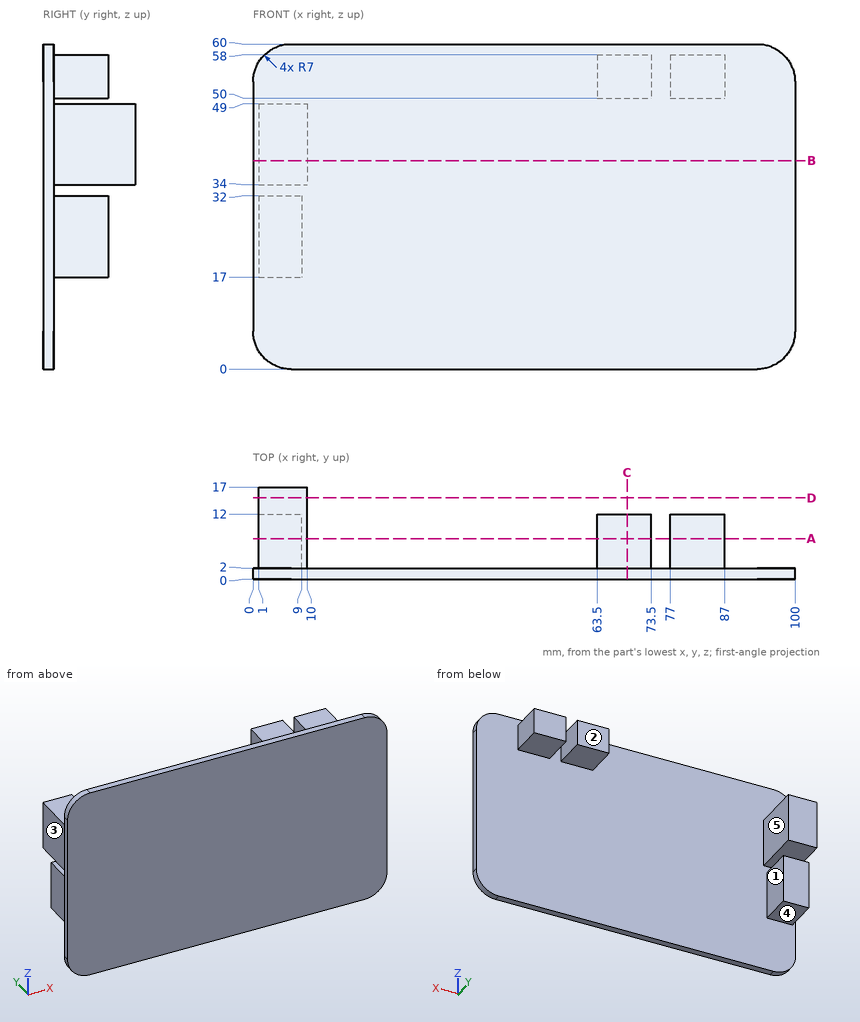
Geometry: see drawing. Coordinates: mm, zero at the bounding-box minimum. A direction names the side the tool comes from. Give positions to 0.01 mm unless a question says otherwise; leave off trailing zeros. Loops run counter-clockwise (first coordinate to the right, second up) from the corner with the lowest first, then second, coordinate; pieces in that order, holes last. Notation, with made-up numbers: (33, 55) -> (68, 55) arc R30 cw to (68, 83) -> close; hole circle Ø9 at (77, 0.25). An arc over 180 degrees is marked (long way). Put each result on its own line as item: value.
1. Set-up query: the marked faces 1, 2, 3, 4 and 5. Return all of +Z, -Z, +X, -X, +Y, -Y with unobstructed straight access to the full face (end or side cutting, diameter ignored); none if empty.
Taken from the geometry:
face 1: -Z, +X, +Y
face 2: +Z, -Z, +X, -X, +Y
face 3: +Z, -Z, -X, +Y
face 4: -Z, +X, -X, +Y
face 5: +Z, -Z, +X, +Y
2. Ray query, line 1 along Y through (x, z) = (17, 53.5); line 2 along X through (y, z) = (14.5, 44); line 3 along X through (y, z) = (11.5, 21). Return the intervals inside material, ascending. Write a range as [from, to].
Taken from the geometry:
line 1: y = [0, 2]
line 2: x = [1, 10]
line 3: x = [1, 9]
3. Cut plane C-C (x = 69). Return the cut outline in (y, z), plus the area to 3 significant figures.
Taken from the geometry:
outline: (0, 0) -> (2, 0) -> (2, 50) -> (12, 50) -> (12, 58) -> (2, 58) -> (2, 60) -> (0, 60) -> close
area: 200 mm2
4. Pin query (flat end, axial travel): P1, Ø7.5, axis at y = 7.5, z = 43.5, coming from the -X side; P2, Ø4, axis at x = 4.5, z = 21, coming from the +Y side; P3, Ø9, axis at x = 5, y = 9, coming from the +Z side; P4, Ø8, axis at x = 49.5, y = 9, coming from the -Z side. Return the tip coordinate at first contact, or that it passes through.
Taken from the geometry:
P1: stops at x = 1
P2: stops at y = 12
P3: stops at z = 49
P4: passes through
5. Cut plane B-B (z = 38.5). Return the cut outline in (x, y).
Taken from the geometry:
outline: (0, 0) -> (100, 0) -> (100, 2) -> (10, 2) -> (10, 17) -> (1, 17) -> (1, 2) -> (0, 2) -> close
6. Cut plane A-A (y = 7.5). Return the cut outline in (x, z).
Taken from the geometry:
outline: (1, 17) -> (9, 17) -> (9, 32) -> (1, 32) -> close; (1, 34) -> (10, 34) -> (10, 49) -> (1, 49) -> close; (63.5, 50) -> (73.5, 50) -> (73.5, 58) -> (63.5, 58) -> close; (77, 50) -> (87, 50) -> (87, 58) -> (77, 58) -> close
7. Cut plane D-D (y = 15). Return the cut outline in (x, z), plus the area to 3 significant figures.
Taken from the geometry:
outline: (1, 34) -> (10, 34) -> (10, 49) -> (1, 49) -> close
area: 135 mm2
